Check sheet for the drawn part. Datum: minimum x, y, z corner. Units: mm. Round coordinates to 2 decimals unless told otherwise and drop trailing zeros. Write each loop counter-clockwise with the first axis right and the second up, starting at its lowest first coordinate (ties: lowest second). Pieces come first, ordered by that corner, then holes. Notation, with made-up numbers: (81, -6) -> (117, -6) arc R29 cw to (117, 29) -> close; hole circle Ø2 at (-11.75, 57.5). An arc over 180 degrees is marked (long way). Use CSV: the item, a comma, the result in double quotes.
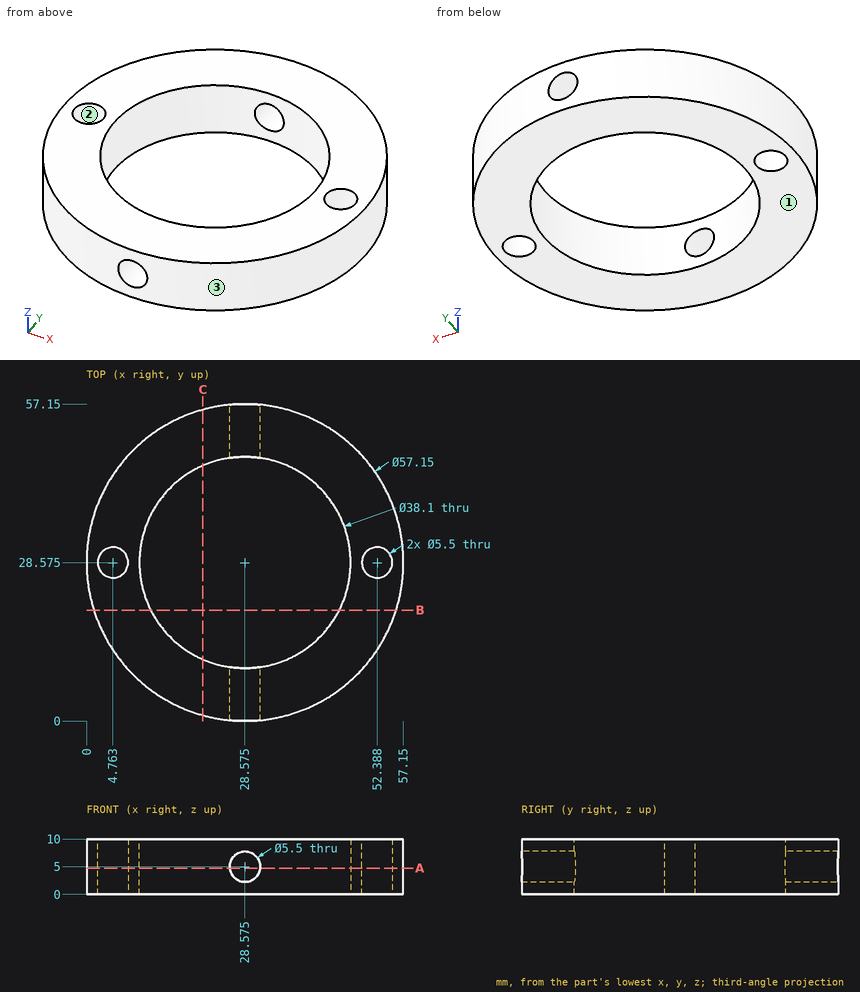
Q1. Section check A-A (z = 4.75). State how many separate pieces and enclosed holes the cut face has, plus the area to 3 significant figures.
Filled in:
separate pieces,"2"
enclosed holes,"2"
area,"1,270 mm²"
Q2. Section check B-B (y = 20). Record the cut outline in (x, z) (1 decimal), plus the area to 3 significant figures.
Filled in:
outline,"(1.3, 0) -> (11.6, 0) -> (11.6, 10) -> (1.3, 10) -> close; (45.6, 0) -> (55.8, 0) -> (55.8, 10) -> (45.6, 10) -> close"
area,"205 mm²"
Q3. Go/stop test with flat-tipped pins: P1, Ø3.5, axis at x = 52.39, y = 28.58, coming from the +Z side; P2, Ø3, axis at y = 28, z = 6, coming from the -X side; P3, Ø2, axis at x = 9, z = 5.5, coming from the +Y side; P4, Ø5, axis at x = 20.5, z = 6, coming from the -Y side. Record where each tip stops, or that it passes through.
Filled in:
P1,"through"
P2,"x = 0"
P3,"y = 50.29"
P4,"y = 0.55"
Q4. Mould release check, pull along Y, two halves, no side actions. Record for the marked faces 1, 2 and 3: released by +Y, released by -Y, zero draft, split by the parting line, or undercut.
Filled in:
face 1,"zero draft"
face 2,"undercut"
face 3,"split by the parting line"
Q5. Material ranges on L1, parallel to X at y = 27, z = 3.5 (1 decimal); L2, parallel to X at y = 16.5, z = 3.75 (1 decimal); L3, parallel to Y at x = 16, z = 9 (1 decimal), recorded low to high.
Filled in:
L1,"0 to 2.5, 7 to 9.6, 47.6 to 50.1, 54.6 to 57.1"
L2,"2.7 to 13.8, 43.3 to 54.5"
L3,"2.9 to 14.3, 42.9 to 54.2"
Q6. Section check C-C (x = 21). Record the cut outline in (y, z) (1 decimal).
Filled in:
outline,"(1, 0) -> (11.1, 0) -> (11.1, 10) -> (1, 10) -> close; (46.1, 0) -> (56.1, 0) -> (56.1, 10) -> (46.1, 10) -> close"
